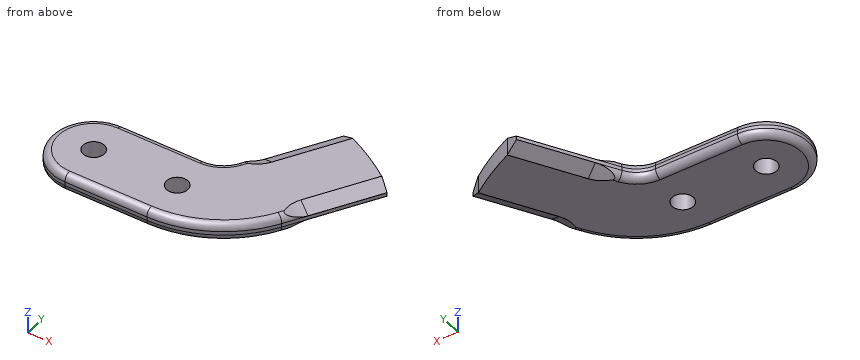
from build123d import *

# Parameters (mm, degrees)
F0_R     = 2.413
F1_DEPTH = 1.9939
F4_R     = 1.5875


with BuildPart() as f1:
    # F0 (on Top) → F1 (new body, symmetric)
    with BuildSketch(Plane.XY):
        with BuildLine():
            Line((18.6904355234, 9.525), (0, 9.525))
            ThreePointArc((0, 9.525), (-9.525, 0), (0, -9.525))
            Line((0, -9.525), (18.6904355234, -9.525))
            ThreePointArc((18.6904355234, -9.525), (31.3904355234, -6.1220452561), (40.6874807795, 3.175))
            ThreePointArc((40.6874807795, 3.175), (39.8367420935, 6.35), (40.6874807795, 9.525))
            Line((40.6874807795, 9.525), (49.0916124422, 24.0813830332))
            ThreePointArc((49.0916124422, 24.0813830332), (43.7515, 27.5320369653), (38.0930898141, 30.4313830332))
            Line((38.0930898141, 30.4313830332), (29.6889581514, 15.875))
            ThreePointArc((29.6889581514, 15.875), (27.3646968374, 13.550738686), (24.1896968374, 12.7))
            ThreePointArc((24.1896968374, 12.7), (21.8654355234, 10.375738686), (18.6904355234, 9.525))
        make_face()
        Circle(F0_R, mode=Mode.SUBTRACT)
        with Locations((19.05, 0)):
            Circle(F0_R, mode=Mode.SUBTRACT)
        with BuildLine():
            Line((35.143388423, 31.6723503567), (24.1896968374, 12.7))
            ThreePointArc((24.1896968374, 12.7), (27.3646968374, 13.550738686), (29.6889581514, 15.875))
            Line((29.6889581514, 15.875), (38.0930898141, 30.4313830332))
            ThreePointArc((38.0930898141, 30.4313830332), (36.6260577586, 31.0704511113), (35.143388423, 31.6723503567))
        make_face()
        with BuildLine():
            ThreePointArc((40.6874807795, 9.525), (39.8367420935, 6.35), (40.6874807795, 3.175))
            Line((40.6874807795, 3.175), (51.6411723651, 22.1473503567))
            ThreePointArc((51.6411723651, 22.1473503567), (50.3785776603, 23.130430044), (49.0916124422, 24.0813830332))
            Line((49.0916124422, 24.0813830332), (40.6874807795, 9.525))
        make_face()
    extrude(amount=F1_DEPTH, both=True)

    # F4
    f4_edges = [f1.edges().sort_by_distance(p)[0] for p in [
        (31.390436, -6.122045, 1.9939),
        (31.390436, -6.122045, -1.9939),
    ]]
    fillet(f4_edges, radius=F4_R)

    # F5: sweep along a path in F0
    with BuildLine(Plane.XY) as f5_path:
        Line((44.5967970303, 41.6961343692), (29.6889581514, 15.875))
        ThreePointArc((29.6889581514, 15.875), (27.3646968374, 13.550738686), (24.1896968374, 12.7))
    # F3 (on line) → F5 (sweep, cut)
    with BuildSketch(Plane(origin=(22.8595967149, 39.5939829508, 0), x_dir=(-0.8660254038, 0.5, 0), z_dir=(0.5, 0.8660254038, 0))):
        Polygon((-17.773891971, 1.9939), (-14.598891971, 0.4064), (-14.598891971, 1.9939), align=None)
        Polygon((-14.598891971, -0.4064), (-17.773891971, -1.9939), (-14.598891971, -1.9939), align=None)
    sweep(path=f5_path.line, mode=Mode.SUBTRACT)

    # F6: sweep along a path in F0
    with BuildLine(Plane.XY) as f6_path:
        Line((55.5953196584, 35.3461343692), (40.6874807795, 9.525))
        ThreePointArc((40.6874807795, 9.525), (39.8367420935, 6.35), (40.6874807795, 3.175))
    # F3 (on line) → F6 (sweep, cut)
    with BuildSketch(Plane(origin=(22.8595967149, 39.5939829508, 0), x_dir=(-0.8660254038, 0.5, 0), z_dir=(0.5, 0.8660254038, 0))):
        Polygon((-33.648891971, 1.9939), (-33.648891971, 0.4213609829), (-30.5038139368, 1.9939), align=None)
        Polygon((-33.648891971, -0.4213609829), (-33.648891971, -1.9939), (-30.5038139368, -1.9939), align=None)
    sweep(path=f6_path.line, mode=Mode.SUBTRACT)


solid = f1.part
Input: part model. Units: mm. Frame: model coordinates. Round coordinates to 2 decimals unless told otherwise and drop trailing zeros. Write each loop counter-clockwise with the first axis right and the second up, starting at its lowest first coordinate (ties: lowest second). Pieces come first, ordered by that corner, then holes.
1) Cut plane A-A (x = 5). Return the cut outline in (y, z) (1 decimal), then the cut area to 3 significant figures.
2) Cut plane C-C (y = 0). Count the separate pieces of the cut face and the enclosed holes in it, then the cut area to 3 significant figures.
3) Contact query for flat-ended pins moving along their axis: P1, Ø4, axis at x = 23.5, y = 15, coming from the +Z side; P2, Ø0.9, axis at x = 13, z = 0, coming from the +Y side (3 decimals); P3, Ø8, axis at x = 42, y = -1, coming from the -Z side. Output: stop coordinate, or through.
4) Ray query, L1, parallel to Y at x = 19.05, z = -0.35; L2, parallel to X at y = -0.5, z = -1.7; L3, parallel to Y at x = 19.05, z = -0.9. Return the intervals inside material, ascending.
5) Cut plane B-B (y = 25). Return the cut outline in (x, z).
Geometry says:
1. outline: (-9.5, -0.4) arc R1.6 ccw to (-7.9, -2) - (7.9, -2) arc R1.6 ccw to (9.5, -0.4) - (9.5, 0.4) arc R1.6 ccw to (7.9, 2) - (-7.9, 2) arc R1.6 ccw to (-9.5, 0.4) - close
1. area: 73.8 mm2
2. separate pieces: 3
2. enclosed holes: 0
2. area: 151 mm2
3. P1: stops at z = 1.27
3. P2: stops at y = 9.525
3. P3: stops at z = -1.67
4. L1: y = -9.52 to -2.41, 2.41 to 9.54
4. L2: x = -8.84 to -2.36, 2.36 to 16.69, 21.41 to 37.23
4. L3: y = -9.44 to -2.41, 2.41 to 9.46
5. outline: (31.29, -0.41) - (34.96, -1.99) - (47.78, -1.99) - (47.78, 1.99) - (34.96, 1.99) - (31.29, 0.41) - close
